Build history of the part. All positions in model axes, mm. A direction names the side the tool comes from. Round coordinates to 2 decimals unless told otherwise and drop trailing zeros. Write each loop counter-clockwise with the first axis right and the second up, starting at its lowest first coordinate (ties: lowest second). Pieces come first, ordered by that corner, then holes. Notation, with made-up numbers: (-22, 65.25) - (-10, 65.25) arc R27 ccw to (-10, 98.25) - close; hole circle Ø5 at (68, -35.75). An arc over 180 degrees is marked (long way). Write each question's results on one line, items separated by ' | '.
from build123d import *

# Parameters (mm, degrees)
FRONT_CONNECTOR_SKETCH_R      = 30
FRONT_CONNECTOR_EXTRUDE_DEPTH = 2
BACK_CONNECTOR_SKETCH_R       = 30
BACK_CONNECTOR_EXTRUDE_DEPTH  = 2
MID_RING_SKETCH_R             = 45
BACK_START                    = 2
BACK_CROSS_CUT_DEPTH          = 48.000004
FRONT_START                   = -50.000001
FRONT_CROSS_CUT_DEPTH         = 48.000002
PIN_HOLE_CUT_DEPTH            = 2
PIN_HOLE_CUT_DEPTH_BACK       = 40
PIN_HOLE_SKETCH_R             = 10


with BuildPart() as part:
    # Front Connector Sketch → Front Connector Extrude (new body)
    with BuildSketch(Plane.XY):
        Circle(FRONT_CONNECTOR_SKETCH_R)
    extrude(amount=-FRONT_CONNECTOR_EXTRUDE_DEPTH)

    # Mid Ring Sketch → section 1 of front_loft
    with BuildSketch(Plane.XY.offset(50), mode=Mode.PRIVATE) as front_loft_s1:
        Circle(MID_RING_SKETCH_R)
    # loft from a face of the part (front_loft)
    loft([part.faces().sort_by_distance((0, 0, 0))[0], front_loft_s1.sketch])



with BuildPart() as body_2:
    # Back Connector Sketch → Back Connector Extrude (new body)
    with BuildSketch(Plane.XY.offset(100)):
        Circle(BACK_CONNECTOR_SKETCH_R)
    extrude(amount=BACK_CONNECTOR_EXTRUDE_DEPTH)


with BuildPart() as part_1:
    add(part.part)

    add(body_2.part)  # back_loft joins it to this body
    # loft up to a face of the part (back_loft)
    loft([Face(Wire([part_1.edges().sort_by_distance((-30.804619767, 32.803588234, 50))[0]])), part_1.faces().sort_by_distance((0, 0, 100))[0]])

    # Cross Cut Sketch → Back Cross Cut (cut)
    with BuildSketch(Plane.XY.offset(50).offset(BACK_START)):
        with BuildLine():
            Line((-12.67766953, 43.177270586), (-12.67766953, 21.5470809))
            ThreePointArc((-12.67766953, 21.5470809), (0, 25), (12.67766953, 21.5470809))
            Line((12.67766953, 21.5470809), (12.67766953, 43.177270586))
            ThreePointArc((12.67766953, 43.177270586), (0, 45), (-12.67766953, 43.177270586))
        make_face()
        with BuildLine():
            Line((-12.67766953, -21.5470809), (-12.67766953, -43.177270586))
            ThreePointArc((-12.67766953, -43.177270586), (0, -45), (12.67766953, -43.177270586))
            Line((12.67766953, -43.177270586), (12.67766953, -21.5470809))
            ThreePointArc((12.67766953, -21.5470809), (0, -25), (-12.67766953, -21.5470809))
        make_face()
        with BuildLine():
            Line((17.67766953, 41.382363393), (17.67766953, 17.67766953))
            Line((17.67766953, 17.67766953), (41.382363393, 17.67766953))
            ThreePointArc((41.382363393, 17.67766953), (31.819805153, 31.819805153), (17.67766953, 41.382363393))
        make_face()
        with BuildLine():
            Line((17.67766953, -17.67766953), (17.67766953, -41.382363393))
            ThreePointArc((17.67766953, -41.382363393), (31.819805153, -31.819805153), (41.382363393, -17.67766953))
            Line((41.382363393, -17.67766953), (17.67766953, -17.67766953))
        make_face()
        with BuildLine():
            Line((-17.67766953, 41.382363393), (-17.67766953, 17.67766953))
            Line((-17.67766953, 17.67766953), (-41.382363393, 17.67766953))
            ThreePointArc((-41.382363393, 17.67766953), (-31.819805153, 31.819805153), (-17.67766953, 41.382363393))
        make_face()
        with BuildLine():
            Line((-17.67766953, -17.67766953), (-17.67766953, -41.382363393))
            ThreePointArc((-17.67766953, -41.382363393), (-31.819805153, -31.819805153), (-41.382363393, -17.67766953))
            Line((-41.382363393, -17.67766953), (-17.67766953, -17.67766953))
        make_face()
        with BuildLine():
            Line((43.177270586, 12.67766953), (21.5470809, 12.67766953))
            ThreePointArc((21.5470809, 12.67766953), (25, 0), (21.5470809, -12.67766953))
            Line((21.5470809, -12.67766953), (43.177270586, -12.67766953))
            ThreePointArc((43.177270586, -12.67766953), (45, 0), (43.177270586, 12.67766953))
        make_face()
        with BuildLine():
            Line((-21.5470809, 12.67766953), (-43.177270586, 12.67766953))
            ThreePointArc((-43.177270586, 12.67766953), (-45, 0), (-43.177270586, -12.67766953))
            Line((-43.177270586, -12.67766953), (-21.5470809, -12.67766953))
            ThreePointArc((-21.5470809, -12.67766953), (-25, 0), (-21.5470809, 12.67766953))
        make_face()
    extrude(amount=BACK_CROSS_CUT_DEPTH, mode=Mode.SUBTRACT)

    # Cross Cut Sketch<2> → Front Cross Cut (cut)
    with BuildSketch(Plane.XY.offset(50).offset(FRONT_START)):
        with BuildLine():
            Line((-12.67766953, 43.177270586), (-12.67766953, 21.5470809))
            ThreePointArc((-12.67766953, 21.5470809), (0, 25), (12.67766953, 21.5470809))
            Line((12.67766953, 21.5470809), (12.67766953, 43.177270586))
            ThreePointArc((12.67766953, 43.177270586), (0, 45), (-12.67766953, 43.177270586))
        make_face()
        with BuildLine():
            Line((-12.67766953, -21.5470809), (-12.67766953, -43.177270586))
            ThreePointArc((-12.67766953, -43.177270586), (0, -45), (12.67766953, -43.177270586))
            Line((12.67766953, -43.177270586), (12.67766953, -21.5470809))
            ThreePointArc((12.67766953, -21.5470809), (0, -25), (-12.67766953, -21.5470809))
        make_face()
        with BuildLine():
            Line((17.67766953, 41.382363393), (17.67766953, 17.67766953))
            Line((17.67766953, 17.67766953), (41.382363393, 17.67766953))
            ThreePointArc((41.382363393, 17.67766953), (31.819805153, 31.819805153), (17.67766953, 41.382363393))
        make_face()
        with BuildLine():
            Line((17.67766953, -17.67766953), (17.67766953, -41.382363393))
            ThreePointArc((17.67766953, -41.382363393), (31.819805153, -31.819805153), (41.382363393, -17.67766953))
            Line((41.382363393, -17.67766953), (17.67766953, -17.67766953))
        make_face()
        with BuildLine():
            Line((-17.67766953, 41.382363393), (-17.67766953, 17.67766953))
            Line((-17.67766953, 17.67766953), (-41.382363393, 17.67766953))
            ThreePointArc((-41.382363393, 17.67766953), (-31.819805153, 31.819805153), (-17.67766953, 41.382363393))
        make_face()
        with BuildLine():
            Line((-17.67766953, -17.67766953), (-17.67766953, -41.382363393))
            ThreePointArc((-17.67766953, -41.382363393), (-31.819805153, -31.819805153), (-41.382363393, -17.67766953))
            Line((-41.382363393, -17.67766953), (-17.67766953, -17.67766953))
        make_face()
        with BuildLine():
            Line((43.177270586, 12.67766953), (21.5470809, 12.67766953))
            ThreePointArc((21.5470809, 12.67766953), (25, 0), (21.5470809, -12.67766953))
            Line((21.5470809, -12.67766953), (43.177270586, -12.67766953))
            ThreePointArc((43.177270586, -12.67766953), (45, 0), (43.177270586, 12.67766953))
        make_face()
        with BuildLine():
            Line((-21.5470809, 12.67766953), (-43.177270586, 12.67766953))
            ThreePointArc((-43.177270586, 12.67766953), (-45, 0), (-43.177270586, -12.67766953))
            Line((-43.177270586, -12.67766953), (-21.5470809, -12.67766953))
            ThreePointArc((-21.5470809, -12.67766953), (-25, 0), (-21.5470809, 12.67766953))
        make_face()
    extrude(amount=FRONT_CROSS_CUT_DEPTH, mode=Mode.SUBTRACT)

    # Pin Hole Sketch → Pin Hole Cut (cut, two sides: drawn at the far end of the back side and taken through both)
    with BuildSketch(Plane.XY.offset(100).offset(-PIN_HOLE_CUT_DEPTH_BACK)):
        Circle(PIN_HOLE_SKETCH_R)
    extrude(amount=PIN_HOLE_CUT_DEPTH + PIN_HOLE_CUT_DEPTH_BACK, mode=Mode.SUBTRACT)


solid = part_1.part
(1) Slice it at B-B, the plane x = 0. Write the cut outline in (y, z), and give its area (3 significant figures).
Worked answers:
outline: (-45, 50) - (-44.4, 48) - (-25, 48) - (-25, 0) - (-30, 0) - (-30, -2) - (30, -2) - (30, 0) - (25, 0) - (25, 48) - (44.4, 48) - (45, 50) - (44.4, 52) - (25, 52) - (25, 100) - (30, 100) - (30, 102) - (10, 102) - (10, 60) - (-10, 60) - (-10, 102) - (-30, 102) - (-30, 100) - (-25, 100) - (-25, 52) - (-44.4, 52) - close | area: 4,560 mm2
(2) Slice it at C-C, the plane z = 34.5. Write the cut outline in (x, y).
Worked answers:
outline: (-38.31, -12.68) arc R40.35 ccw to (-36.27, -17.68) - (-17.68, -17.68) - (-17.68, -36.27) arc R40.35 ccw to (-12.68, -38.31) - (-12.68, -21.55) arc R25 ccw to (12.68, -21.55) - (12.68, -38.31) arc R40.35 ccw to (17.68, -36.27) - (17.68, -17.68) - (36.27, -17.68) arc R40.35 ccw to (38.31, -12.68) - (21.55, -12.68) arc R25 ccw to (21.55, 12.68) - (38.31, 12.68) arc R40.35 ccw to (36.27, 17.68) - (17.68, 17.68) - (17.68, 36.27) arc R40.35 ccw to (12.68, 38.31) - (12.68, 21.55) arc R25 ccw to (-12.68, 21.55) - (-12.68, 38.31) arc R40.35 ccw to (-17.68, 36.27) - (-17.68, 17.68) - (-36.27, 17.68) arc R40.35 ccw to (-38.31, 12.68) - (-21.55, 12.68) arc R25 ccw to (-21.55, -12.68) - close
(3) Drill centre lines: probe 1 along Z at (x, y) = (28.5, 1); probe 2 along Y at (x, z) = (0, 89); probe 3 along Y at (x, z) = (-31, 35.5). Where is each one in solid material? Low to high. Write a range as [from, to].
Worked answers:
probe 1: z = [-2, 0], [48, 52], [100, 102] | probe 2: y = [-25, -10], [10, 25] | probe 3: y = [-17.68, -12.68], [12.68, 17.68]
(4) Flat gauge pins, fed straight in: pin 1 Ø7 at (y, z) = (-26.5, 21) entering from +X; pin 2 Ø3 at (x, z) = (34.5, 41) entering from -Y; pin 3 Ø3 at (x, y) = (-21, 28.5) entering from +Z. Where does each tip first touch, or does it go through?
Worked answers:
pin 1: stops at x = 17.68 | pin 2: stops at y = -17.68 | pin 3: stops at z = 52
(5) Two-plate mould, pull along Y, no slides. Class faces 5 (the cylindrical face through (-25, 0, 76)), 6 (the flat face through (-17.678, -26, 70)), 7 (the conical face through (-14.461, -32.216, 17.709)): released by +Y, released by -Y, zero draft, split by the parting line, or undercut.
Worked answers:
face 5: undercut | face 6: zero draft | face 7: split by the parting line
(6) Tool access for faces 1 (the flat face through (-26, 17.678, 29)), 2 (the flat face through (30, -12.678, 29)), 3 (the flat face through (-12.678, -30, 29)), 4 (the flat face through (20, 20, 100)): list every direction of +Z, -Z, +X, -X, +Y, -Y with a clear straight run to the whole face (end or side of a thin tool).
Worked answers:
face 1: -X, +Y | face 2: +X | face 3: -Y | face 4: +X, +Y
